Could you check a few things on this model? Use its own coordinates, in mm. A direction names the side the tool comes from. Give positions to 0.01 mm unless a question says otherwise; leave off trailing zeros. Order: outer loops, then holes, each group sorted by start corner. A loop starts at its lowest first (then second) coordinate and runs counter-clockwise, first axis right, second up.
(1) If I drill on probe 1 along X at (y, z) = (7.5, 1.15); probe 2 along Y at (x, z) = (24.75, 1.3); probe 3 along X at (y, z) = (-8.5, 1.3), over which ranges is the centre line in solid material (lowest first)?
(2) On a 3-axis mill with a long thin cutter (end or side, diameter ignored), from which of +Z, -Z, +X, -X, +Y, -Y can I reach the whole of each face in a straight line? I mean faces 1 (the flat face through (14.75, -4, 1)), 2 (the flat face through (22.75, -1, 1)), 3 (the flat face through (4, -10, 0)), 4 (the flat face through (19.75, -11, 1)), 5 (the cylindrical face through (-18.7, 4.3, 1)). Say none if no direction works.
(3) Imagine slicing it at C-C, the plane x = 5.5. Write out the boundary of the cut face in (y, z), then the cut area to 3 significant figures.
(4) Imagine slicing it at A-A, the plane z = 1.25. State how many separate pieces and enclosed holes the cut face has, then the cut area to 3 significant figures.
(5) Imagine slicing it at D-D, the plane y = -5.8. Write out the boundary of the cut face in (x, z), then the cut area to 3 significant figures.
(6) Imagine slicing it at B-B, the plane y = -0.5. Write out the boundary of the cut face in (x, z), then the cut area to 3 significant figures.
(7) Will these pins go through, and if not, where does the flat tip stop? pin 1 (1 mm diameter, centred on x = -21.5, z = 0.5, fed in from -Y); pin 2 (5 mm diameter, centred on x = 24.75, y = -24.25, fed in from -Z); pin 3 (0.6 mm diameter, centred on y = 7.5, z = 1, fed in from +X); pin 4 (1 mm diameter, centred on y = 1, z = 1, fed in from +X).
(8) If we mould it in two halves opening along Y, with no side actions, what happens to faces 6 (the flat face through (0.97, -20.1, 0.99)), 7 (the flat face through (-19.75, -9, 1)), 8 (the flat face through (8.409, -10.293, 0.986)), 9 (the cylindrical face through (30.27, -26.6, 0.99))? For each: released by +Y, released by -Y, zero draft, split by the parting line, or undercut.
Autodesk Inventor part; units mm, degrees
ref_plane "YZ Plane" through (0, 0, 0) normal (1, 0, 0) x (0, 1, 0)
ref_plane "XZ Plane" through (0, 0, 0) normal (0, 1, 0) x (-1, 0, 0)
ref_plane "XY Plane" through (0, 0, 0) normal (0, 0, 1) x (1, 0, 0)
sketch "スケッチ1" plane through (0, 0, 0) normal (0, 0, 1) x (1, 0, 0)
  line L0 (-19.75, 25.75) -> (19.75, 25.75) construction
  line L1 (19.75, 25.75) -> (19.75, -25.75) construction
  line L2 (19.75, -25.75) -> (-19.75, -25.75) construction
  line L3 (-19.75, -25.75) -> (-19.75, 25.75) construction
  line L4 (-19.75, 25.75) -> (19.75, -25.75) construction
  line L5 (19.75, 25.75) -> (-19.75, -25.75) construction
  circle A0 centre (24.75, -24.25) radius 1.55
  circle A1 centre (-7.25, -4.25) radius 2.25
  line L6 (0, 25.75) -> (0, -25.75) construction
  line L7 (-19.75, 3.25) -> (-22.75, 3.25)
  line L8 (-22.75, 3.25) -> (-22.75, -4.75)
  arc A2 (-19.75, 3.25) -> (-19.75, 5.35) centre (-19.75, 4.3) ccw
  line L9 (-22.75, -0.75) -> (-19.75, -0.75) construction
  line L10 (-19.75, -4.75) -> (-22.75, -4.75)
  arc A3 (-19.75, -6.85) -> (-19.75, -4.75) centre (-19.75, -5.8) ccw
  line L11 (-19.75, 5.35) -> (-19.75, 9.25)
  line L12 (-19.75, 9.25) -> (19.75, 9.25)
  line L13 (22.75, 3.25) -> (22.75, -4.75)
  arc A4 (19.75, 5.35) -> (19.75, 3.25) centre (19.75, 4.3) ccw
  line L14 (19.75, -4.75) -> (22.75, -4.75)
  arc A5 (19.75, -4.75) -> (19.75, -6.85) centre (19.75, -5.8) ccw
  line L15 (19.75, 5.35) -> (19.75, 9.25)
  line L16 (19.75, 3.25) -> (22.75, 3.25)
  arc A6 (22.2819, -29.7189) -> (27.2181, -18.7811) centre (24.75, -24.25) ccw
  line L17 (-19.75, -6.85) -> (-19.75, -10.75)
  line L18 (-19.75, -10.75) -> (22.2819, -29.7189)
  line L19 (19.75, -6.85) -> (19.75, -15.4108)
  line L20 (19.75, -15.4108) -> (27.2181, -18.7811)
  circle A7 centre (-7.25, -4.25) radius 6 construction
  circle A8 centre (24.75, -24.25) radius 6 construction
  line L21 (2.75, 5.25) -> (14.75, 5.25)
  line L22 (14.75, 5.25) -> (14.75, -13.1543)
  line L23 (14.75, -13.1543) -> (2.75, -7.7388)
  line L24 (2.75, -7.7388) -> (2.75, 5.25)
  point P0 (0, 0)
  dimension "d0" = 39.5
  dimension "d1" = 51.5
  dimension "d2" = 3.1
  dimension "d3" = 4.5
  dimension "d4" = 32
  dimension "d5" = 20
  dimension "d6" = 3
  dimension "d7" = 1.05
  dimension "d8" = 8
  dimension "d9" = 26.5
  dimension "d11" = 30
  dimension "d12" = 12.5
  dimension "d13" = 6
  dimension "d14" = 12
  dimension "d19" = 12
  dimension "d20" = 12
  dimension "d21" = 4
  dimension "d22" = 5
  dimension "d24" = 4
extrude "押し出し1" add sketch "スケッチ1" along normal blind 2
fillet "フィレット1" radius 1 1 edges at (19.75, -15.4108, 1)
fillet "フィレット2" radius 1 4 edges at (2.75, 5.25, 1) (14.75, 5.25, 1) (2.75, -7.7388, 1) (14.75, -13.1543, 1)
equation "\"d24\" = d21"
properties part number "付け根_メインフレーム_1" material "アルミニウム 2014-T4"
Answer block:
1. probe 1: x = -19.75 to 19.75
1. probe 2: y = -30.25 to -25.8, -22.7 to -17.67
1. probe 3: x = -19.75 to 4.44, 14.75 to 19.75
2. face 1: +Z, -Z
2. face 2: +Z, -Z, +X, +Y
2. face 3: -Z, +X, -X, +Y, -Y
2. face 4: +Z, -Z, +X
2. face 5: +Z, -Z, -X
3. outline: (-22.15, 0) - (-8.98, 0) - (-8.98, 2) - (-22.15, 2) - close; (5.25, 0) - (9.25, 0) - (9.25, 2) - (5.25, 2) - close
3. area: 34.3 mm2
4. separate pieces: 1
4. enclosed holes: 3
4. area: 1,090 mm2
5. outline: (-18.7, 0) - (-8.88, 0) - (-8.88, 2) - (-18.7, 2) - close; (-5.62, 0) - (2.75, 0) - (2.75, 2) - (-5.62, 2) - close; (14.75, 0) - (18.7, 0) - (18.7, 2) - (14.75, 2) - close
5. area: 44.3 mm2
6. outline: (-22.75, 0) - (2.75, 0) - (2.75, 2) - (-22.75, 2) - close; (14.75, 0) - (22.75, 0) - (22.75, 2) - (14.75, 2) - close
6. area: 67.0 mm2
7. pin 1: stops at y = -4.75
7. pin 2: stops at z = 0
7. pin 3: stops at x = 19.75
7. pin 4: stops at x = 22.75
8. face 6: released by -Y
8. face 7: zero draft
8. face 8: undercut
8. face 9: split by the parting line
